For this review, use the dimensioned drawing (mm, ordinates from the lowest corner) and the shaded views. A direction names the side the tool comes from. Coordinates: 2 decimals unless noted, no trailing zeros. Loops run counter-clockwise (first coordinate to the right, second up) from the corner with the lowest first, then second, coordinate; pieces in that order, holes last. Notation, with made-up numbers: M 6.25,85 L 24.25,85 A35 ccw 24.25,122 Z; hole C 8.25,49.25 d9. An arc over 180 degrees is marked long. One line per item, written item: value.
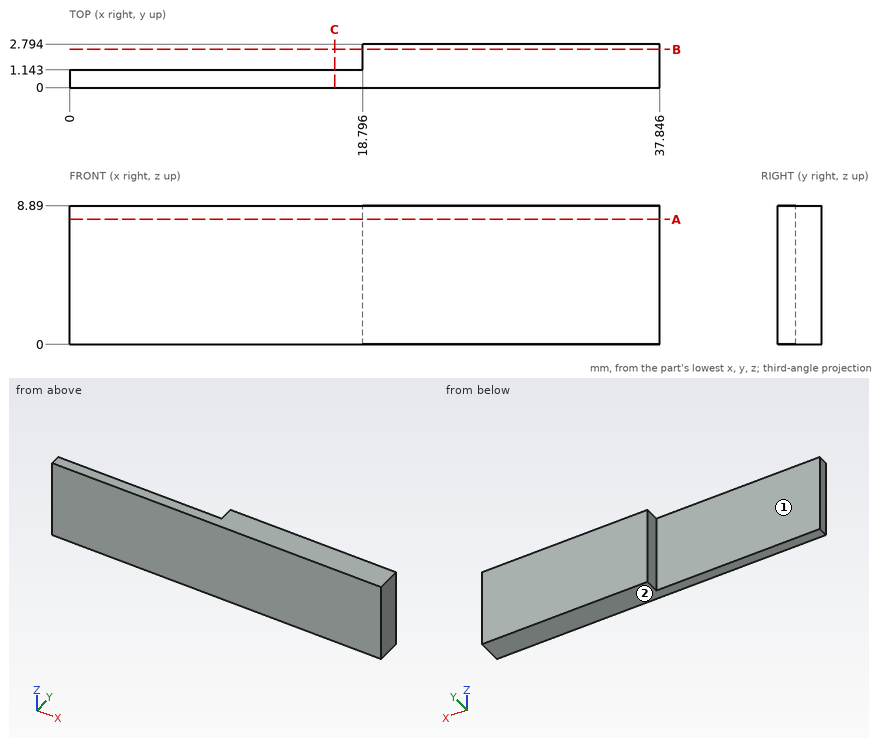
(1) Insertion check: pin 1 (2.5 mm diameter, centred on x = 14, z = 5.5, fed in from +Y). The pin has a flat end and moves straight along its axis. Give the tip position at first contact, or say it passes through.
Reply:
pin 1: stops at y = 1.14
(2) We need section C-C on x = 17. State the section outline as (y, z) points.
Reply:
outline: M 0,0 L 1.14,0 L 1.14,8.89 L 0,8.89 Z
(3) Tool access review of the marked faces 1 and 2: name each direction out of +Z, -Z, +X, -X, +Y, -Y from which nothing blocks a thin tool from reaching the whole face with its end or side.
Reply:
face 1: +Z, -Z, -X, +Y
face 2: -Z, +X, -X, +Y, -Y
(4) We need section A-A on z = 8. State the section outline as (x, y) points, then the cut area to 3 significant figures.
Reply:
outline: M 0,0 L 37.85,0 L 37.85,2.79 L 18.8,2.79 L 18.8,1.14 L 0,1.14 Z
area: 74.7 mm2
(5) We need section B-B on y = 2.45. State the section outline as (x, z) points.
Reply:
outline: M 18.8,0 L 37.85,0 L 37.85,8.89 L 18.8,8.89 Z
(6) To check wall thickness, follow line 1 along X through (y, z) = (2.2, 8.75); line 2 along Y through (x, z) = (6.5, 0.75). State the ranges of each line that lie inside material, in increasing order. Write a range as [from, to].
Reply:
line 1: x = [18.8, 37.85]
line 2: y = [0, 1.14]
